The listing builds one solid part. Answer for the finished solid, in the listing's coordinates (mm). A direction names the side the tool comes from. Round coordinates to 2 decimals unless told otherwise and drop trailing zeros. Loops run counter-clockwise (first coordinate to the right, second up) from the corner with the lowest first, then second, coordinate; pieces in that order, holes last. Notation, with made-up numbers: (-16.75, 10) -> (11.25, 10) arc R34 ccw to (11.25, 45) -> close; hole circle Ø10 at (-11, 50.5). An arc over 180 degrees is marked (long way). Write each question's results on one line, items separated by ' | '. Start each with the question number.
(1) Determine the mould class of faces 4 (the face through (-11, 4, -14)), 5 (the face through (-17.5, 3, 0)), 6 (the face through (3, 12, 3)) for opening direction X: released by +X, released by -X, zero draft, split by the parting line, or undercut.
(2) Flat-ended cylindrical pins translate along their axes: pin 1 (4 mm diameter, centred on x = 6, y = 10, fed in from +Z); pin 2 (2 mm diameter, centred on x = -12.5, z = -11.5, fed in from -Y); pin 3 (6 mm diameter, centred on x = 12.37, z = -12.37, fed in from +Y). Find the tip coordinate at first contact, or state that the pin passes through.
(3) The part is cut by section D-D (y = 5.75). Determine the outline of the cut face in (x, z), plus the area to 3 significant figures.
(4) The part is cut by section A-A (z = 0). Determine the outline of the cut face in (x, y).
(5) For faces 1 (the face through (15.168, 3.451, 15.238)), 2 (the face through (-11, 4, 11)), 3 (the face through (12.932, 9.535, 5.362)), determine the directions among +Z, -Z, +X, -X, +Y, -Y from which every point of the face is accessible in a straight line to the end or side of a thin tool.
(6) The part is cut by section B-B (x = 0). Determine the outline of the cut face in (y, z), plus the area to 3 significant figures.
(7) Straight lines are drawn through the part: probe 1 along X at (y, z) = (7.25, 0); probe 2 along X at (y, z) = (6, 0); probe 3 along X at (y, z) = (1.25, -13). For each, find the intervals that lie inside material, in ascending order.
(8) The part is cut by section C-C (x = 5.5). Determine the outline of the cut face in (y, z), plus the area to 3 significant figures.
```python
from build123d import *

# Parameters (mm, degrees)
SKETCH_5_R          = 4
SKETCH_5_R_2        = 1.7
EXTRUDE_2_DEPTH     = 12
SKETCH_7_W          = 35
SKETCH_7_H          = 35
SKETCH_7_R          = 14
CUT_EXTRUDE_4_DEPTH = 5
SKETCH_8_R          = 3.25
CUT_EXTRUDE_5_DEPTH = 4


with BuildPart() as part:
    # Эскиз5 → Бобышка-Вытянуть2 (new body)
    with BuildSketch(Plane(origin=(0, 0, 0), x_dir=(1, 0, 0), z_dir=(0, 1, 0))):
        with BuildLine():
            Line((-12.489995997, -17.5), (12.489995997, -17.5))
            ThreePointArc((12.489995997, -17.5), (15.202795796, -15.202795796), (17.5, -12.489995997))
            Line((17.5, -12.489995997), (17.5, 12.489995997))
            ThreePointArc((17.5, 12.489995997), (15.202795796, 15.202795796), (12.489995997, 17.5))
            Line((12.489995997, 17.5), (-12.489995997, 17.5))
            ThreePointArc((-12.489995997, 17.5), (-15.202795796, 15.202795796), (-17.5, 12.489995997))
            Line((-17.5, 12.489995997), (-17.5, -12.489995997))
            ThreePointArc((-17.5, -12.489995997), (-15.202795796, -15.202795796), (-12.489995997, -17.5))
        make_face()
        Circle(SKETCH_5_R, mode=Mode.SUBTRACT)
        with Locations((-12.374368671, 12.374368671)):
            Circle(SKETCH_5_R_2, mode=Mode.SUBTRACT)
        with Locations((12.374368671, 12.374368671)):
            Circle(SKETCH_5_R_2, mode=Mode.SUBTRACT)
        with Locations((12.374368671, -12.374368671)):
            Circle(SKETCH_5_R_2, mode=Mode.SUBTRACT)
        with Locations((-12.374368671, -12.374368671)):
            Circle(SKETCH_5_R_2, mode=Mode.SUBTRACT)
    extrude(amount=EXTRUDE_2_DEPTH)

    # Эскиз7 → Вырез-Вытянуть4 (cut)
    with BuildSketch(Plane(origin=(0, 12, 0), x_dir=(1, 0, 0), z_dir=(0, 1, 0))):
        Rectangle(SKETCH_7_W, SKETCH_7_H)
        Circle(SKETCH_7_R, mode=Mode.SUBTRACT)
    extrude(amount=-CUT_EXTRUDE_4_DEPTH, mode=Mode.SUBTRACT)

    # Эскиз8 → Вырез-Вытянуть5 (cut)
    with BuildSketch(Plane.XZ):
        with Locations((-12.374368671, 12.374368671)):
            Circle(SKETCH_8_R)
        with Locations((12.374368671, 12.374368671)):
            Circle(SKETCH_8_R)
        with Locations((12.374368671, -12.374368671)):
            Circle(SKETCH_8_R)
        with Locations((-12.374368671, -12.374368671)):
            Circle(SKETCH_8_R)
    extrude(amount=-CUT_EXTRUDE_5_DEPTH, mode=Mode.SUBTRACT)


solid = part.part
```
Checked values:
1) face 4: undercut | face 5: released by -X | face 6: zero draft
2) pin 1: stops at z = 13.42 | pin 2: stops at y = 4 | pin 3: stops at y = 7
3) outline: (-17.5, -12.49) arc R21.5 ccw to (-12.49, -17.5) -> (12.49, -17.5) arc R21.5 ccw to (17.5, -12.49) -> (17.5, 12.49) arc R21.5 ccw to (12.49, 17.5) -> (-12.49, 17.5) arc R21.5 ccw to (-17.5, 12.49) -> close; hole circle Ø3.4 at (-12.37, -12.37); hole circle Ø3.4 at (-12.37, 12.37); hole circle Ø8 at (0, 0); hole circle Ø3.4 at (12.37, -12.37); hole circle Ø3.4 at (12.37, 12.37) | area: 1,090 mm2
4) outline: (-17.5, 0) -> (-4, 0) -> (-4, 12) -> (-14, 12) -> (-14, 7) -> (-17.5, 7) -> close; (4, 0) -> (17.5, 0) -> (17.5, 7) -> (14, 7) -> (14, 12) -> (4, 12) -> close
5) face 1: +Z, +X, +Y, -Y | face 2: -Y | face 3: +Y
6) outline: (0, -17.5) -> (7, -17.5) -> (7, -14) -> (12, -14) -> (12, -4) -> (0, -4) -> close; (0, 4) -> (12, 4) -> (12, 14) -> (7, 14) -> (7, 17.5) -> (0, 17.5) -> close | area: 289 mm2
7) probe 1: x = -14 to -4, 4 to 14 | probe 2: x = -17.5 to -4, 4 to 17.5 | probe 3: x = -17.12 to -15.56, -9.19 to 9.19, 15.56 to 17.12
8) outline: (0, -17.5) -> (7, -17.5) -> (7, -12.87) -> (12, -12.87) -> (12, 12.87) -> (7, 12.87) -> (7, 17.5) -> (0, 17.5) -> close | area: 374 mm2
